Geometry: final body of the model. Coordinates: model frame, mm. A direction names the side the tool comes from. Coordinates: 2 decimals unless noted, no trailing zeros. Loops run counter-clockwise (first coordinate to the right, second up) from the corner with the lowest first, then second, coordinate; pieces in that order, holes last. Notation, with made-up numbers: (-13, 40.25) - (34, 40.25) arc R10 cw to (34, 48.25) - close; hole circle Ø7 at (-17.75, 14.25). An arc over 180 degrees is marked (long way). Put each result on its own line as item: value. Start each with the question number.
1) Contact query for flat-ended pins moving along their axis: pin 1 Ø1.6 at (y, z) = (1.5, 49.5) entering from -X; pin 2 Ø1.6 at (y, z) = (1, 17) entering from +X. Output: stop coordinate, or through.
2) Section B-B on x = 0. Output: boundary loops of the cut face in (y, z) (3 decimals), and give its area (3 significant figures).
3) Section C-C on y = 1.9. Output: boundary loops of the cut face in (x, z), and give its area (3 significant figures).
4) Reachability of faces 4 (the flat face through (-26, 2, -50.8)), 5 (the flat face through (6.604, 2, 45)), 6 (the flat face through (12.7, 2, 14)), 7 (the flat face through (-9, 3.175, -18)) from +Z, -Z, +X, -X, +Y, -Y: full face, straight path, thin tool, end or side. Return the list, or none.
5) Material intervals for line 1 along X through (y, z) = (2.45, -63.5); line 2 along X through (y, z) = (2.55, -17); line 3 along Z through (x, y) = (-1, 1.1), sorted ascending. Write a range as from..to.
6) Section A-A on z = -63.5. Output: boundary loops of the cut face in (x, y) (3 decimals), and give its area (3 significant figures).
7) Section D-D on x = -25.4. Output: boundary loops of the cut face in (y, z) (3 decimals), and give its area (3 significant figures).
8) Draft query along Z for faces 1 (the cylindrical face through (-0.15, 1.61, -36.32)), 2 (the flat face through (-12.7, 2, 12)), 3 (the flat face through (0, 2, 76.2)). Return one class per face: +Z half, -Z half, draft (parallel to the pull), parting line (faces both ways), or undercut.
```python
from build123d import *

# Parameters (mm, degrees)
SKETCH1_W           = 25.4
SKETCH1_H           = 25.4
BOSS_EXTRUDE1_DEPTH = 3.175
SKETCH2_R           = 3.3734375
CUT_EXTRUDE1_DEPTH  = 3.175
FILLET1_R           = 2.54


with BuildPart() as part:
    # Sketch1 → Boss-Extrude1 (new body)
    with BuildSketch(Plane(origin=(0, 0, 0), x_dir=(1, 0, 0), z_dir=(0, 1, 0))):
        with Locations((-25.4, 63.5)):
            Rectangle(SKETCH1_W, SKETCH1_H)
        Polygon((-12.7, -76.2), (12.7, -76.2), (12.7, 50.8), (12.7, 76.2), (-12.7, 76.2), (-12.7, 50.8), align=None)
        with Locations((25.4, 63.5)):
            Rectangle(SKETCH1_W, SKETCH1_H)
    extrude(amount=BOSS_EXTRUDE1_DEPTH)

    # Sketch2 → Cut-Extrude1 (cut)
    with BuildSketch(Plane(origin=(0, 3.175, 0), x_dir=(1, 0, 0), z_dir=(0, 1, 0))):
        with Locations(Location((-25.4, 63.5, 0), (0, 0, 270))):
            Circle(SKETCH2_R)
        with Locations(Location((25.4, 63.5, 0), (0, 0, 270))):
            Circle(SKETCH2_R)
        with BuildLine():
            Line((6.604, 29.718), (6.604, 6.35))
            ThreePointArc((6.604, 6.35), (0, -0.254), (-6.604, 6.35))
            Line((-6.604, 6.35), (-6.604, 29.718))
            ThreePointArc((-6.604, 29.718), (0, 36.322), (6.604, 29.718))
        make_face()
        with BuildLine():
            Line((6.604, -33.782), (6.604, -57.15))
            ThreePointArc((6.604, -57.15), (0, -63.754), (-6.604, -57.15))
            Line((-6.604, -57.15), (-6.604, -33.782))
            ThreePointArc((-6.604, -33.782), (0, -27.178), (6.604, -33.782))
        make_face()
    extrude(amount=-CUT_EXTRUDE1_DEPTH, mode=Mode.SUBTRACT)

    # Fillet1
    fillet1_edges = [part.edges().sort_by_distance(p)[0] for p in [
        (38.1, 1.5875, -76.2),
        (38.1, 1.5875, -50.8),
        (12.7, 1.5875, -50.8),
        (12.7, 1.5875, 76.2),
        (-12.7, 1.5875, 76.2),
        (-12.7, 1.5875, -50.8),
        (-38.1, 1.5875, -50.8),
        (-38.1, 1.5875, -76.2),
    ]]
    fillet(fillet1_edges, radius=FILLET1_R)


solid = part.part
```
Answer block:
1. pin 1: stops at x = -12.7
1. pin 2: stops at x = 12.7
2. outline: (0, -76.2) - (3.175, -76.2) - (3.175, -36.322) - (0, -36.322) - close; (0, 0.254) - (3.175, 0.254) - (3.175, 27.178) - (0, 27.178) - close; (0, 63.754) - (3.175, 63.754) - (3.175, 76.2) - (0, 76.2) - close
2. area: 252 mm²
3. outline: (-38.1, -73.66) arc R2.54 ccw to (-35.56, -76.2) - (35.56, -76.2) arc R2.54 ccw to (38.1, -73.66) - (38.1, -53.34) arc R2.54 ccw to (35.56, -50.8) - (15.24, -50.8) arc R2.54 cw to (12.7, -48.26) - (12.7, 73.66) arc R2.54 ccw to (10.16, 76.2) - (-10.16, 76.2) arc R2.54 ccw to (-12.7, 73.66) - (-12.7, -48.26) arc R2.54 cw to (-15.24, -50.8) - (-35.56, -50.8) arc R2.54 ccw to (-38.1, -53.34) - close; hole circle Ø6.75 at (-25.4, -63.5); hole (-6.6, -29.72) arc R6.6 ccw to (6.6, -29.72) - (6.6, -6.35) arc R6.6 ccw to (-6.6, -6.35) - close; hole (-6.6, 33.78) arc R6.6 ccw to (6.6, 33.78) - (6.6, 57.15) arc R6.6 ccw to (-6.6, 57.15) - close; hole circle Ø6.75 at (25.4, -63.5)
3. area: 4,190 mm²
4. face 4: +Z, -X, +Y, -Y
4. face 5: +Y, -Y
4. face 6: +Z, +X, +Y, -Y
4. face 7: +Z, -Z, +X, -X, +Y
5. line 1: x = -38.1..-28.77, -22.03..22.03, 28.77..38.1
5. line 2: x = -12.7..-6.6, 6.6..12.7
5. line 3: z = -76.2..-36.25, 0.18..27.25, 63.68..76.2
6. outline: (-38.1, 0) - (-28.773, 0) - (-28.773, 3.175) - (-38.1, 3.175) - close; (-22.027, 0) - (22.027, 0) - (22.027, 3.175) - (-22.027, 3.175) - close; (28.773, 0) - (38.1, 0) - (38.1, 3.175) - (28.773, 3.175) - close
6. area: 199 mm²
7. outline: (0, -76.2) - (3.175, -76.2) - (3.175, -66.873) - (0, -66.873) - close; (0, -60.127) - (3.175, -60.127) - (3.175, -50.8) - (0, -50.8) - close
7. area: 59.2 mm²
8. face 1: undercut
8. face 2: draft
8. face 3: +Z half
